Part model, mm, in its own coordinate system. Face numbers are marked on the shaded views. A direction names the side the tool comes from. Coordinates: 2 decimals unless noted, no trailing zeros. Order: outer loops, then holes, each group sorted by start corner. A loop starts at its lowest first (then second) coordinate and runs counter-clockwise, first axis right, second up.
from build123d import *

# Parameters (mm, degrees)
SKETCH2_R          = 5
CUT_EXTRUDE1_DEPTH = 24.454743657
SKETCH3_R          = 2
CUT_EXTRUDE2_DEPTH = 24.454743657


with BuildPart() as part:
    # Sketch1 → Revolve1 (revolve)
    with BuildSketch(Plane(origin=(0, 0, 0), x_dir=(0, 0, -1), z_dir=(1, 0, 0)), mode=Mode.PRIVATE) as revolve1_sk:
        Polygon((0, 0), (0, 11.5), (-9.5, 11.5), (-9.5, 6), (-12, 6), (-12, 11.5), (-13, 11.5), (-13, 12.75), (-15, 12.75), (-15, 0), align=None)
    revolve(revolve1_sk.sketch.rotate(Axis((0, 0, 15), (0, 0, -1)), 90), axis=Axis((0, 0, 15), (0, 0, -1)))

    # Sketch2 → Cut-Extrude1 (cut, through all)
    with BuildSketch(Plane.XY.offset(15)):
        Circle(SKETCH2_R)
    extrude(amount=-CUT_EXTRUDE1_DEPTH, mode=Mode.SUBTRACT)

    # Sketch3 → Cut-Extrude2 (cut, through all)
    with BuildSketch(Plane.XY.offset(15)):
        with Locations((0, 8.875)):
            Circle(SKETCH3_R)
        with Locations((8.875, 0)):
            Circle(SKETCH3_R)
        with Locations((0, -8.875)):
            Circle(SKETCH3_R)
        with Locations((-8.875, 0)):
            Circle(SKETCH3_R)
    extrude(amount=-CUT_EXTRUDE2_DEPTH, mode=Mode.SUBTRACT)


solid = part.part
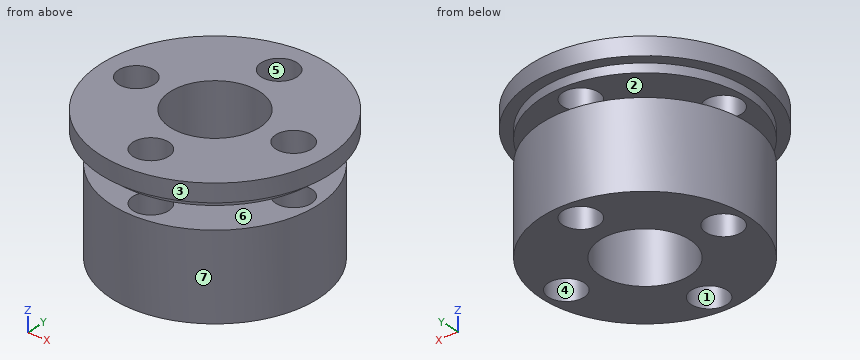
Q1. Wall check: line 1 along Y through (x, z) = (0, 12.7) (3 decimals); line 2 along Y through (x, z) = (0, 11); line 3 along Z through (x, y) = (-8.75, 6). Give the ranges that are in metal, low to high.
Results list:
line 1: y = -11.5 to -10.875, -6.875 to -5, 5 to 6.875, 10.875 to 11.5
line 2: y = -6 to -5, 5 to 6
line 3: z = 0 to 9.5, 12 to 15
Q2. Cut at A-A on y = -4. Write the cut outline in (x, z).
Results list:
outline: (-12.11, 13) - (-10.78, 13) - (-10.78, 12) - (-4.47, 12) - (-4.47, 9.5) - (-10.78, 9.5) - (-10.78, 0) - (-3, 0) - (-3, 15) - (-12.11, 15) - close; (3, 0) - (10.78, 0) - (10.78, 9.5) - (4.47, 9.5) - (4.47, 12) - (10.78, 12) - (10.78, 13) - (12.11, 13) - (12.11, 15) - (3, 15) - close
Q3. Cut at D-D on x = 0. Count the separate pieces of the cut face and the enclosed holes in it, and give its area (3 significant figures).
Results list:
separate pieces: 6
enclosed holes: 0
area: 72.5 mm2
Q4. Which spindle directions (+Z, -Z, +X, -X, +Y, -Y) get a long thin tool onto all of the face, cutting with end or side? Do the marked faces 5, 6 and 7. Say none if no direction does.
Results list:
face 5: +Z, -Z
face 6: none
face 7: -Z
Q5. Pin check, flat tips, straight feed: pin 1 Ø4.5 at (x, y) = (0, -8.875) entering from +Z; pin 2 Ø6 at (y, z) = (-10, 5) entering from +X; pin 3 Ø6 at (y, z) = (2.5, 11) entering from +X; pin 4 Ø4 at (x, z) = (-1, 5) entering from -Y. Stop position of each tip, or through.
Results list:
pin 1: stops at z = 15
pin 2: stops at x = 9.12
pin 3: stops at x = 12.75
pin 4: stops at y = -11.5
Q6. Cut at C-C on y = -7.75. Write the cut outline in (x, z), and give its area (3 significant figures).
Results list:
outline: (-10.12, 13) - (-8.5, 13) - (-8.5, 12) - (-1.65, 12) - (-1.65, 15) - (-10.12, 15) - close; (-8.5, 0) - (-1.65, 0) - (-1.65, 9.5) - (-8.5, 9.5) - close; (1.65, 0) - (8.5, 0) - (8.5, 9.5) - (1.65, 9.5) - close; (1.65, 12) - (8.5, 12) - (8.5, 13) - (10.12, 13) - (10.12, 15) - (1.65, 15) - close
area: 178 mm2
Q7. Cut at B-B on x = 10. Write the cut outline in (y, z), and give its area (3 significant figures).
Results list:
outline: (-7.91, 13) - (-5.68, 13) - (-5.68, 12) - (-1.65, 12) - (-1.65, 15) - (-7.91, 15) - close; (-5.68, 0) - (-1.65, 0) - (-1.65, 9.5) - (-5.68, 9.5) - close; (1.65, 0) - (5.68, 0) - (5.68, 9.5) - (1.65, 9.5) - close; (1.65, 12) - (5.68, 12) - (5.68, 13) - (7.91, 13) - (7.91, 15) - (1.65, 15) - close
area: 110 mm2
Q8. Mould opens along Y. For the marked faces 1, 2, 3 and 4 say: pulls with the +Y half, pulls with the -Y half, needs draft (parallel to the pull), parting line crosses it, or undercut.
Results list:
face 1: undercut
face 2: needs draft
face 3: parting line crosses it
face 4: undercut
